Model file for the job. Use its own axes, mm. Round coordinates to 2 decimals unless told otherwise and drop trailing zeros. Loops run counter-clockwise (first coordinate to the right, second up) from the corner with the lowest first, then second, coordinate; pieces in that order, holes last. Notation, with made-up numbers: (51.25, 23) -> (59.25, 23) arc R23 cw to (59.25, 40) -> close; hole circle Ø5 at (-19.75, 72). An arc over 180 degrees is marked (long way). Use a Markdown table: item, result.
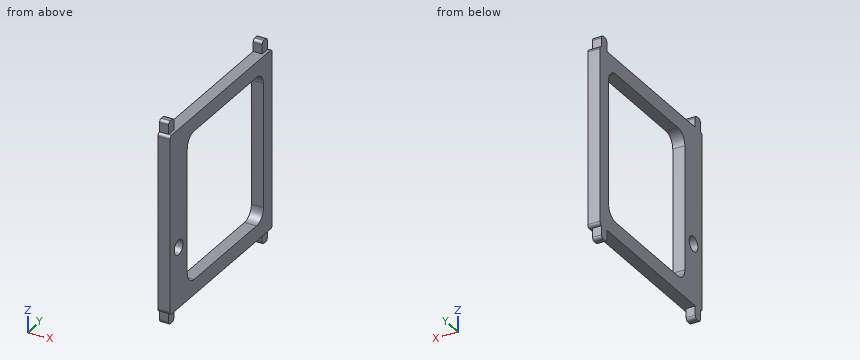
from build123d import *

# Parameters (mm, degrees)
F0_R     = 2.5
F0_W     = 3
F0_H     = 4
F1_DEPTH = 4
F2_W     = 3
F2_H     = 4
F3_DEPTH = 1
F4_R     = 4
F5_R     = 0.99999


# Not quite as in the source:
# - a fillet or chamfer is up to 0.001 mm smaller than in the source, because OpenCascade refuses the exact size


with BuildPart() as f1:
    # F0 (on Right) → F1 (new body)
    with BuildSketch(Plane.YZ):
        Polygon((-28.5, 29.5), (-29.5, 29.5), (-29.5, -29.5), (-28.5, -29.5), (-25.5, -29.5), (25.5, -29.5), (28.5, -29.5), (29.5, -29.5), (29.5, 29.5), (28.5, 29.5), (25.5, 29.5), (-25.5, 29.5), align=None)
        with Locations((-24.5, -9.5)):
            Circle(F0_R, mode=Mode.SUBTRACT)
        Polygon((19.5, -24.5), (-19.5, -24.5), (-19.5, 24.5), (19.5, 24.5), (24.5, 24.5), (24.5, -24.5), align=None, mode=Mode.SUBTRACT)
        with Locations((-27, 31.5)):
            Rectangle(F0_W, F0_H)
        with Locations((27, 31.5)):
            Rectangle(F0_W, F0_H)
        with Locations((-27, -31.5)):
            Rectangle(F0_W, F0_H)
        with Locations((27, -31.5)):
            Rectangle(F0_W, F0_H)
    extrude(amount=F1_DEPTH)

    # F2 (on face) → F3 (cut)
    with BuildSketch(Plane.YZ.offset(4)):
        with Locations((-27, 31.5)):
            Rectangle(F2_W, F2_H)
        with Locations((27, 31.5)):
            Rectangle(F2_W, F2_H)
        with Locations((-27, -31.5)):
            Rectangle(F2_W, F2_H)
        with Locations((27, -31.5)):
            Rectangle(F2_W, F2_H)
    extrude(amount=-F3_DEPTH, mode=Mode.SUBTRACT)

    # F4
    f4_edges = [f1.edges().sort_by_distance(p)[0] for p in [
        (2, -19.5, 24.5),
        (2, 24.5, 24.5),
        (2, 24.5, -24.5),
        (2, -19.5, -24.5),
    ]]
    fillet(f4_edges, radius=F4_R)

    # F5 (radius 1 in the source; OpenCascade refuses exactly that, so slightly less here)
    f5_edges = [f1.edges().sort_by_distance(p)[0] for p in [
        (1.5, -28.5, 33.5),
        (2, -29.5, 29.5),
        (1.5, -25.5, 33.5),
        (1.5, 25.5, 33.5),
        (1.5, 28.5, 33.5),
        (2, 29.5, 29.5),
        (1.5, -25.5, -33.5),
        (1.5, -28.5, -33.5),
        (2, -29.5, -29.5),
        (1.5, 25.5, -33.5),
        (1.5, 28.5, -33.5),
        (2, 29.5, -29.5),
    ]]
    fillet(f5_edges, radius=F5_R)


solid = f1.part
Q1. Drill centre lines: L1, parallel to Z at x = 2.35, y = -24.5; L2, parallel to Y at x = 1.75, z = 18; L3, parallel to Z at x = 2.2, y = -13. Where is each one in solid material? Low to high. Write a range as from..to.
Results list:
| item | result |
|---|---|
| L1 | z = -29.5..-12, -7..29.5 |
| L2 | y = -29.5..-19.5, 24.5..29.5 |
| L3 | z = -29.5..-24.5, 24.5..29.5 |
Q2. Band-saw the part on A-A, the plane z = 1.5. Give the cut face in (x, y).
Results list:
| item | result |
|---|---|
| outline | (0, -29.5) -> (4, -29.5) -> (4, -19.5) -> (0, -19.5) -> close; (0, 24.5) -> (4, 24.5) -> (4, 29.5) -> (0, 29.5) -> close |
Q3. Band-saw the part on C-C, the plane z = -9.5. Give the cut face in (x, y), plus the area to 3 significant figures.
Results list:
| item | result |
|---|---|
| outline | (0, -29.5) -> (4, -29.5) -> (4, -27) -> (0, -27) -> close; (0, -22) -> (4, -22) -> (4, -19.5) -> (0, -19.5) -> close; (0, 24.5) -> (4, 24.5) -> (4, 29.5) -> (0, 29.5) -> close |
| area | 40.0 mm² |
Q4. Flat gauge pins, fed straight in: pin 1 (1.5 mm diameter, centred on y = -26.5, z = 32.5, fed in from +X); pin 2 (0.9 mm diameter, centred on x = 2, z = 31, fed in from +Y); pin 3 (2 mm diameter, centred on x = 3.5, y = -17, fed in from -Z). Where does each tip first touch, or does it go through?
Results list:
| item | result |
|---|---|
| pin 1 | stops at x = 3 |
| pin 2 | stops at y = 28.5 |
| pin 3 | stops at z = -29.5 |
Q5. Band-saw the part on D-D, the plane x = 0.65. Give the number of separate pieces and of enclosed holes in the cut face, plus the area to 3 significant figures.
Results list:
| item | result |
|---|---|
| separate pieces | 1 |
| enclosed holes | 2 |
| area | 1,360 mm² |
Q6. Band-saw the part on B-B, the plane y = -3. Give the cut face in (x, z).
Results list:
| item | result |
|---|---|
| outline | (0, -29.5) -> (4, -29.5) -> (4, -24.5) -> (0, -24.5) -> close; (0, 24.5) -> (4, 24.5) -> (4, 29.5) -> (0, 29.5) -> close |
